Source: CAD feature listing. Evaluate the final solid. Frame: model axes, mm. A direction names the side the tool comes from. Give positions to 0.01 mm unless a question says otherwise; leave off trailing zeros. Order: outer loops, then holes, each group sorted by start corner. A loop starts at its lowest first (then second) coordinate and runs counter-clockwise, first axis right, second up.
from build123d import *

# Parameters (mm, degrees)
EXTRUDE_1_DEPTH     = 80
SKETCH_2_R          = 1.75
CUT_EXTRUDE_1_DEPTH = 81.847077869


with BuildPart() as part:
    # ｽｹｯﾁ1 → ﾎﾞｽ - 押し出し1 (new body)
    with BuildSketch(Plane.XY):
        Polygon((0, 0), (-7, 0), (-7, 6.5), (-8.5, 6.5), (-8.5, -1.5), (8.5, -1.5), (8.5, 6.5), (7, 6.5), (7, 0), align=None)
    extrude(amount=EXTRUDE_1_DEPTH)

    # ｽｹｯﾁ2 → ｶｯﾄ - 押し出し1 (cut, through all)
    with BuildSketch(Plane.XZ.offset(1.5)):
        with Locations(Location((0, 50, 0), (0, 0, 270))):
            Circle(SKETCH_2_R)
        with Locations(Location((0, 60, 0), (0, 0, 270))):
            Circle(SKETCH_2_R)
    extrude(amount=-CUT_EXTRUDE_1_DEPTH, mode=Mode.SUBTRACT)


solid = part.part
1) Pull-direction query (Z, two-part tool) for faces 3 (the face through (8, 6.5, 39)), 4 (the face through (0, -1, 0)), 5 (the face through (-0.67, -0.76, 48.383)), 6 (the face through (-0.67, -0.76, 58.383)); classes: +Z half, -Z half, draft (parallel to the pull), parting line (faces both ways), or undercut.
Checks:
face 3: draft
face 4: -Z half
face 5: undercut
face 6: undercut
2) Section query A-A on y = 4.5. Output: boundary loops of the cut face in (x, z), and give its area (3 significant figures).
Checks:
outline: (-8.5, 0) - (-7, 0) - (-7, 80) - (-8.5, 80) - close; (7, 0) - (8.5, 0) - (8.5, 80) - (7, 80) - close
area: 240 mm2
3) Reachability of faces 1 (the face through (-8, 6.5, 39)), 2 (the face through (7, 3, 39)) from +Z, -Z, +X, -X, +Y, -Y: full face, straight path, thin tool, end or side. Return the list, or none.
Checks:
face 1: +Z, -Z, +X, -X, +Y
face 2: +Z, -Z, +Y
4) Ray query, L1, parallel to X at y = 1, z = 48; L2, parallel to X at y = -0.9, z = 60; L3, parallel to Y at x = -6.25, z = 16.5. Return the intervals inside material, ascending.
Checks:
L1: x = -8.5 to -7, 7 to 8.5
L2: x = -8.5 to -1.75, 1.75 to 8.5
L3: y = -1.5 to 0
5) First-contact query: pin 1 Ø7 at (x, z) = (-3, 29.5) entering from +Y. Flat tip, straight axial feed; report the tip coordinate or a pass-through.
Checks:
pin 1: stops at y = 0
6) Section query C-C on z = 60. Output: boundary loops of the cut face in (x, y).
Checks:
outline: (-8.5, -1.5) - (-1.75, -1.5) - (-1.75, 0) - (-7, 0) - (-7, 6.5) - (-8.5, 6.5) - close; (1.75, -1.5) - (8.5, -1.5) - (8.5, 6.5) - (7, 6.5) - (7, 0) - (1.75, 0) - close
7) Section query D-D on z = 10. Output: boundary loops of the cut face in (x, y).
Checks:
outline: (-8.5, -1.5) - (8.5, -1.5) - (8.5, 6.5) - (7, 6.5) - (7, 0) - (-7, 0) - (-7, 6.5) - (-8.5, 6.5) - close
8) Section query B-B on x = 0. Output: boundary loops of the cut face in (y, z).
Checks:
outline: (-1.5, 0) - (0, 0) - (0, 48.25) - (-1.5, 48.25) - close; (-1.5, 51.75) - (0, 51.75) - (0, 58.25) - (-1.5, 58.25) - close; (-1.5, 61.75) - (0, 61.75) - (0, 80) - (-1.5, 80) - close
